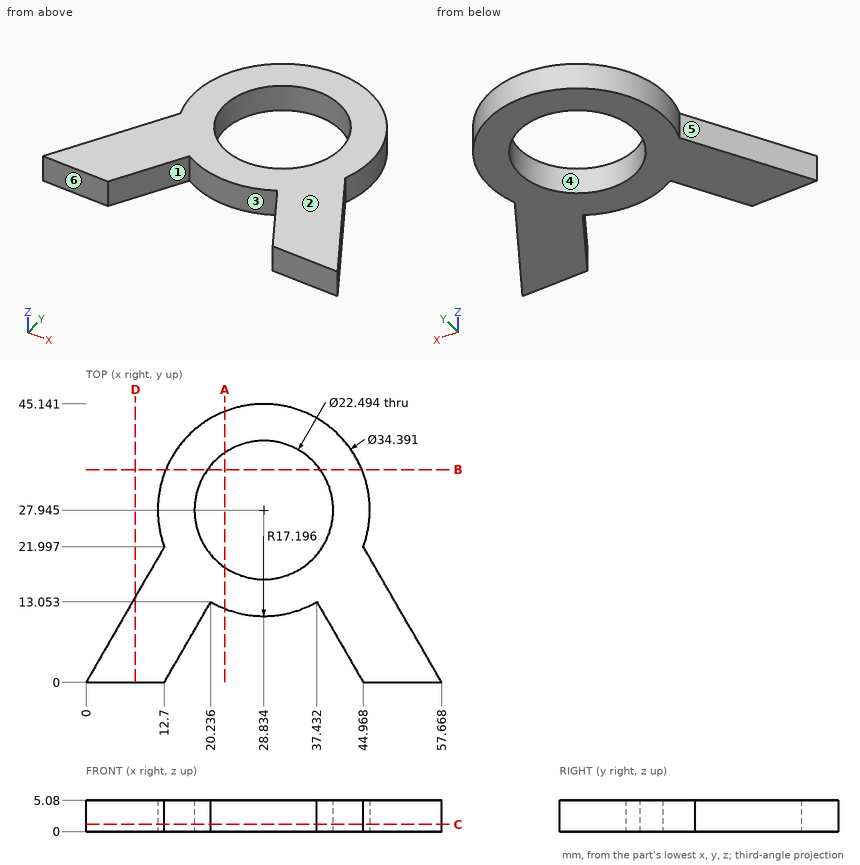
Design review of the part shown in the three views and the two pictorial views. Dimensions are in mm from the part's minimum x, y and z. A direction names the side the tool comes from. Coordinates: 2 decimals unless noted, no trailing zeros. Order: outer loops, then holes, each group sorted by start corner. A loop starts at its lowest first (then second) coordinate and runs counter-clockwise, first axis right, second up.
Item 1: Take a section at A-A, the plane x = 22.5. Write out the cut boundary in (y, z).
Item 2: The part is to be moulded in two halves that separate along X. For the marked faces 3, 4, 5 and 6, say which applies: pulls with the +X half, pulls with the -X half, needs draft (parallel to the pull), parting line crosses it, or undercut.
Item 3: For line 1 (X direction, y = 27.5, z = 4.55) (1 decimal); line 2 (Y direction, x = 38.5, z = 4.55) (1 decimal); line 3 (Y direction, x = 24, z = 0.6), list the stretches that pass through material, from the lowest coordinate up.
Item 4: Take a section at C-C, the plane z = 1.2. Write out the cut boundary in (x, y) (1 decimal).
Item 5: For pin 1 Ø1.5 at (y, z) = (29, 4) entering from -X; pin 2 Ø13.5 at (x, y) = (28.83, 27.95) entering from +Z; pin 3 Ø2 at (y, z) = (38.5, 2) entering from -X, all flat-tipped, find the tip position at first contact; note any pin that passes through.
Item 6: For the marked faces 1 and 2, list the 3-axis set-ups (+Z, -Z, +X, -X, +Y, -Y) from which the entire face can be reached by the end or side of a thin tool; tool diameter is ignored.
Item 7: Take a section at D-D, the plane x = 8. Write out the cut boundary in (y, z).
Item 8: Take a section at B-B, the plane y = 34.5. Write out the cut boundary in (x, z) (1 decimal).
The answers:
1. outline: (11.96, 0) - (18.65, 0) - (18.65, 5.08) - (11.96, 5.08) - close; (37.24, 0) - (43.93, 0) - (43.93, 5.08) - (37.24, 5.08) - close
2. face 3: undercut
2. face 4: undercut
2. face 5: pulls with the -X half
2. face 6: needs draft
3. line 1: x = 11.6 to 17.6, 40.1 to 46
3. line 2: y = 11.2 to 22.2, 33.7 to 42.2
3. line 3: y = 11.44 to 17.79, 38.1 to 44.45
4. outline: (0, 0) - (12.7, 0) - (20.2, 13.1) arc R17.2 ccw to (37.4, 13.1) - (45, 0) - (57.7, 0) - (45, 22) arc R17.2 ccw (long way) to (12.7, 22) - close; hole circle Ø22.5 at (28.8, 27.9)
5. pin 1: stops at x = 11.64
5. pin 2: passes through
5. pin 3: stops at x = 14.54
6. face 1: +Z, -Z, -Y
6. face 2: +Z, +X, -X, +Y, -Y
7. outline: (0, 0) - (13.86, 0) - (13.86, 5.08) - (0, 5.08) - close
8. outline: (12.9, 0) - (19.7, 0) - (19.7, 5.1) - (12.9, 5.1) - close; (38, 0) - (44.7, 0) - (44.7, 5.1) - (38, 5.1) - close
